Build history of the part. All positions in model axes, mm. A direction names the side the tool comes from. Coordinates: 2 decimals unless noted, no trailing zeros. Write each loop counter-clockwise with the first axis right and the second up, starting at its lowest first coordinate (ties: lowest second). Pieces come first, ordered by that corner, then holes.
```python
from build123d import *

# Parameters (mm, degrees)
SKETCH1_R           = 15.24
CUT_EXTRUDE1_START  = -3.81
CUT_EXTRUDE1_DEPTH  = 3.81
SKETCH17_R          = 33.401
CUT_EXTRUDE4_DEPTH  = 0.762
BOSS_EXTRUDE1_DEPTH = 0.762


with BuildPart() as part:
    # Sweep1: sweep along a path in Sketch14
    with BuildLine(Plane(origin=(0, 0, 0), x_dir=(0, 0, -1), z_dir=(1, 0, 0))) as sweep1_path:
        Line((35.814, 0), (35.814, 3.81))
    # Sketch1 → Sweep1 (sweep)
    with BuildSketch(Plane(origin=(0, 0, 0), x_dir=(1, 0, 0), z_dir=(0, 1, 0))):
        with BuildLine():
            Line((35.147120935, 6.5405), (37.341023687, 6.5405))
            ThreePointArc((37.341023687, 6.5405), (26.806064521, 26.806064521), (6.5405, 37.341023687))
            Line((6.5405, 37.341023687), (6.5405, 35.147120935))
            ThreePointArc((6.5405, 35.147120935), (0, 35.7505), (-6.5405, 35.147120935))
            Line((-6.5405, 35.147120935), (-6.5405, 37.341023687))
            ThreePointArc((-6.5405, 37.341023687), (-26.806064521, 26.806064521), (-37.341023687, 6.5405))
            Line((-37.341023687, 6.5405), (-35.147120935, 6.5405))
            ThreePointArc((-35.147120935, 6.5405), (-35.7505, 0), (-35.147120935, -6.5405))
            Line((-35.147120935, -6.5405), (-37.341023687, -6.5405))
            ThreePointArc((-37.341023687, -6.5405), (-26.806064521, -26.806064521), (-6.5405, -37.341023687))
            Line((-6.5405, -37.341023687), (-6.5405, -35.147120935))
            ThreePointArc((-6.5405, -35.147120935), (0, -35.7505), (6.5405, -35.147120935))
            Line((6.5405, -35.147120935), (6.5405, -37.341023687))
            ThreePointArc((6.5405, -37.341023687), (26.806064521, -26.806064521), (37.341023687, -6.5405))
            Line((37.341023687, -6.5405), (35.147120935, -6.5405))
            ThreePointArc((35.147120935, -6.5405), (35.7505, 0), (35.147120935, 6.5405))
        make_face()
        Circle(SKETCH1_R, mode=Mode.SUBTRACT)
    sweep(path=sweep1_path.line)

    # Sketch2 → Cut-Extrude1 (cut)
    with BuildSketch(Plane.XZ.offset(CUT_EXTRUDE1_START)):
        with BuildLine():
            Line((16.256, 37.235541419), (16.256, 11.763792756))
            ThreePointArc((16.256, 11.763792756), (-19.089751858, -6.182696014), (20.066, 0))
            Line((20.066, 0), (20.066, 35.328440735))
            ThreePointArc((20.066, 35.328440735), (18.186016036, 36.331968038), (16.256, 37.235541419))
        make_face()
    extrude(amount=CUT_EXTRUDE1_DEPTH, mode=Mode.SUBTRACT)

    # Sketch17 → Cut-Extrude4 (cut)
    with BuildSketch(Plane.XZ.offset(-3.81)):
        Circle(SKETCH17_R)
    extrude(amount=CUT_EXTRUDE4_DEPTH, mode=Mode.SUBTRACT)

    # Sketch19 → Boss-Extrude1 (add)
    with BuildSketch(Plane.XZ):
        with BuildLine():
            Line((16.256, 11.763792756), (16.256, 15.155628954))
            ThreePointArc((16.256, 15.155628954), (-18.375594526, -12.501525939), (20.066, 9.555431387))
            Line((20.066, 9.555431387), (20.066, 0))
            ThreePointArc((20.066, 0), (-19.089751858, -6.182696014), (16.256, 11.763792756))
        make_face()
    extrude(amount=BOSS_EXTRUDE1_DEPTH)


solid = part.part
```
1. Saw through at A-A on x = 0. List the corners of the cut face in (y, z) (1 decimal).
Computed values:
outline: (-0.8, -22.2) - (0, -22.2) - (0, -35.8) - (3.8, -35.8) - (3.8, -33.4) - (3, -33.4) - (3, -20.1) - (-0.8, -20.1) - close; (-0.8, 20.1) - (3, 20.1) - (3, 33.4) - (3.8, 33.4) - (3.8, 35.8) - (0, 35.8) - (0, 22.2) - (-0.8, 22.2) - close
2. Saw through at C-C on y = 1.4. List the corners of the cut face in (x, z), plus the area to 3 significant figures.
Computed values:
outline: (-37.34, -6.54) arc R37.91 ccw to (-6.54, -37.34) - (-6.54, -35.15) arc R35.75 ccw to (6.54, -35.15) - (6.54, -37.34) arc R37.91 ccw to (37.34, -6.54) - (35.15, -6.54) arc R35.75 ccw to (35.15, 6.54) - (37.34, 6.54) arc R37.91 ccw to (20.07, 32.16) - (20.07, 0) arc R20.07 cw (long way) to (16.26, 11.76) - (16.26, 34.25) arc R37.91 ccw to (6.54, 37.34) - (6.54, 35.15) arc R35.75 ccw to (-6.54, 35.15) - (-6.54, 37.34) arc R37.91 ccw to (-37.34, 6.54) - (-35.15, 6.54) arc R35.75 ccw to (-35.15, -6.54) - close
area: 3,040 mm2
3. Probe line 1 along Z through (x, y) = (0, 0.85); line 2 along X through (y, z) = (3.4, 0); line 3 along X through (y, z) = (-0.5, 0) (3 decimals). List the from-to ranges inside material, lowest first.
Computed values:
line 1: z = -35.75 to -20.07, 20.07 to 35.75
line 2: x = -35.75 to -33.4, 33.4 to 35.75
line 3: x = -22.225 to -20.066, 20.066 to 22.225
4. 3-axis set-ups, long thin cutter, end or side, ignore diameter. For faces 1 (the face through (-36, 2, 6.541)), 2 (the face through (36, 2, -6.541)), 3 (the face through (6.54, 2, 36)), 4 (the face through (-16, 0, -17)): which of +Z, -Z, +X, -X, +Y, -Y reach the whole face in a straight line?
Computed values:
face 1: -X, +Y, -Y
face 2: +X, +Y, -Y
face 3: +Z, +Y, -Y
face 4: -Y
5. Flat gauge pins, fed straight in: pin 1 (1 mm diameter, centred on x = -6, y = 3.5, fed in from -Z); pin 2 (1.9 mm diameter, centred on y = 1.5, z = 8.5, fed in from -X); pin 3 (2 mm diameter, centred on x = 13, y = 0.5, fed in from -Z). Where does each tip first touch, or does it go through?
Computed values:
pin 1: stops at z = -35.32
pin 2: stops at x = -37.15
pin 3: stops at z = -35.96
6. Saw through at D-D on x = 25. List the corners of the cut face in (y, z).
Computed values:
outline: (0, -28.5) - (3.81, -28.5) - (3.81, -22.15) - (3.05, -22.15) - (3.05, 22.15) - (3.81, 22.15) - (3.81, 28.5) - (0, 28.5) - close
7. Mould opens along Z. For faces 5 (the face through (-6.54, 2, 36)), 6 (the face through (-18.882, -0.376, -11.722)), 7 (the face through (-27.03, 1.93, 26.58)), 8 (the face through (-19.391, 3.434, -27.196)) say: +Z half, -Z half, draft (parallel to the pull), parting line (faces both ways), or undercut.
Computed values:
face 5: draft
face 6: parting line
face 7: +Z half
face 8: undercut
8. Saw through at B-B on z = -1.5. List the corners of the cut face in (x, y).
Computed values:
outline: (-35.72, 0) - (-22.17, 0) - (-22.17, -0.76) - (-20.01, -0.76) - (-20.01, 3.05) - (-33.37, 3.05) - (-33.37, 3.81) - (-35.72, 3.81) - close; (20.01, -0.76) - (22.17, -0.76) - (22.17, 0) - (35.72, 0) - (35.72, 3.81) - (33.37, 3.81) - (33.37, 3.05) - (20.01, 3.05) - close
